from build123d import *

# Parameters (mm, degrees)
F0_R         = 38.1
F0_R_2       = 31.75
F1_DEPTH     = 123.825
F2_R         = 5.08
F3_R         = 38.1
F3_R_2       = 31.75
F1_FACE_R    = 38.1
F1_FACE_R_2  = 31.75
F1_FACE1_R   = 33.02
F1_FACE1_R_2 = 31.75
F4_DEPTH     = 4.445


with BuildPart() as f1:
    # F0 (on Top) → F1 (new body)
    with BuildSketch(Plane.XY):
        Circle(F0_R)
        Circle(F0_R_2, mode=Mode.SUBTRACT)
    extrude(amount=F1_DEPTH)

    # F2
    f2_edges = [f1.edges().sort_by_distance(p)[0] for p in [
        (-38.1, 0, 123.825),
    ]]
    fillet(f2_edges, radius=F2_R)

    # F3 (on face) + F1_face (on face) + F0 (on Top) + F1_face1 (on face) → F4 (join, symmetric)
    with BuildSketch(Plane.XY):
        Circle(F3_R)
        Circle(F3_R_2, mode=Mode.SUBTRACT)
        Circle(F3_R_2)
    with BuildSketch(Plane(origin=(0, 0, 0), x_dir=(1, 0, 0), z_dir=(0, 0, -1))):
        Circle(F1_FACE_R)
        Circle(F1_FACE_R_2, mode=Mode.SUBTRACT)
    with BuildSketch(Plane.XY):
        Circle(F0_R)
        Circle(F0_R_2, mode=Mode.SUBTRACT)
    with BuildSketch(Plane.XY.offset(123.825)):
        Circle(F1_FACE1_R)
        Circle(F1_FACE1_R_2, mode=Mode.SUBTRACT)
    extrude(amount=F4_DEPTH, both=True, dir=(0, 0, 1))


solid = f1.part
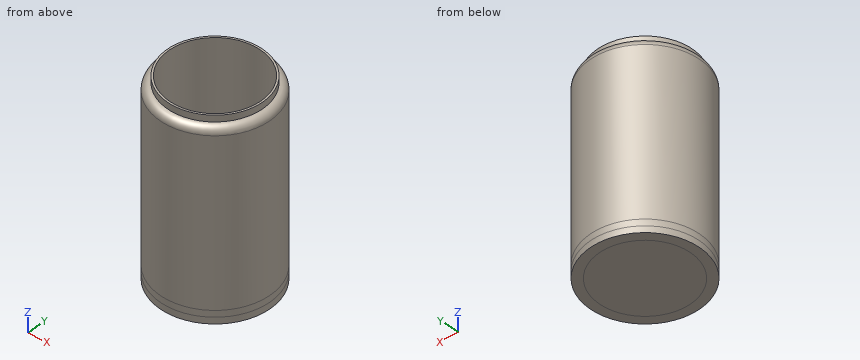
Build history of the part. All positions in model axes, mm. Coordinates: 2 decimals unless noted, no trailing zeros. Write each loop counter-clockwise with the first axis right and the second up, starting at its lowest first coordinate (ties: lowest second). Pieces come first, ordered by that corner, then holes.
(1) Drill centre lines: line 1 (Y direction, x = 0, z = 32.5); line 2 (Z direction, x = -18, y = 17.5) (3 decimals); line 3 (Y direction, x = 18, z = 10.5). Where is each one in solid material? Low to high.
(2) Cut at A-A on y = 0. List the corners of the cut face in (x, z) (3 decimals), and give its area (3 significant figures).
(3) Cut at B-B on z = 101.5. List the corners of the cut face in (x, y).
(4) Pin check, flat tips, straight feed: pin 1 Ø12 at (y, z) = (-6, 90.5) entering from -X; pin 2 Ø1.5 at (x, z) = (27.5, 102) entering from -Y; pin 3 Ø2 at (x, z) = (-29.5, 30) entering from +Y; pin 4 Ø8 at (y, z) = (-10, 74.5) entering from +X. Stop position of each tip, or through.
Working result:
1. line 1: y = -38.1 to -31.75, 31.75 to 38.1
1. line 2: z = -4.445 to 4.445
1. line 3: y = -33.58 to -26.15, 26.15 to 33.58
2. outline: (-38.1, -4.445) - (38.1, -4.445) - (38.1, 118.745) arc R5.08 ccw to (33.02, 123.825) - (33.02, 128.27) - (31.75, 128.27) - (31.75, 4.445) - (-31.75, 4.445) - (-31.75, 128.27) - (-33.02, 128.27) - (-33.02, 123.825) arc R5.08 ccw to (-38.1, 118.745) - close
2. area: 2,190 mm2
3. outline: circle Ø76.2 at (0, 0); hole circle Ø63.5 at (0, 0)
4. pin 1: stops at x = -38.1
4. pin 2: stops at y = -27.13
4. pin 3: stops at y = 25.29
4. pin 4: stops at x = 37.62
